Part print with two shaded views. Sizes in mm from the minimum x, y, z corner. A direction names the side the tool comes from. Give positions to 0.01 mm unless a question says otherwise; leave off trailing zeros. Order: outer loops, then holes, each group sorted by start corner. A loop starts at its lowest first (then second) coordinate and runs counter-clockwise, first axis right, second up. Notation, with made-up numbers: M 35.5,39 L 85.5,39 A12 ccw 85.5,51 Z; hole C -37.5,87.25 d9. An arc over 180 degrees is marked long. Return JSON: item names as keys, results as strings.
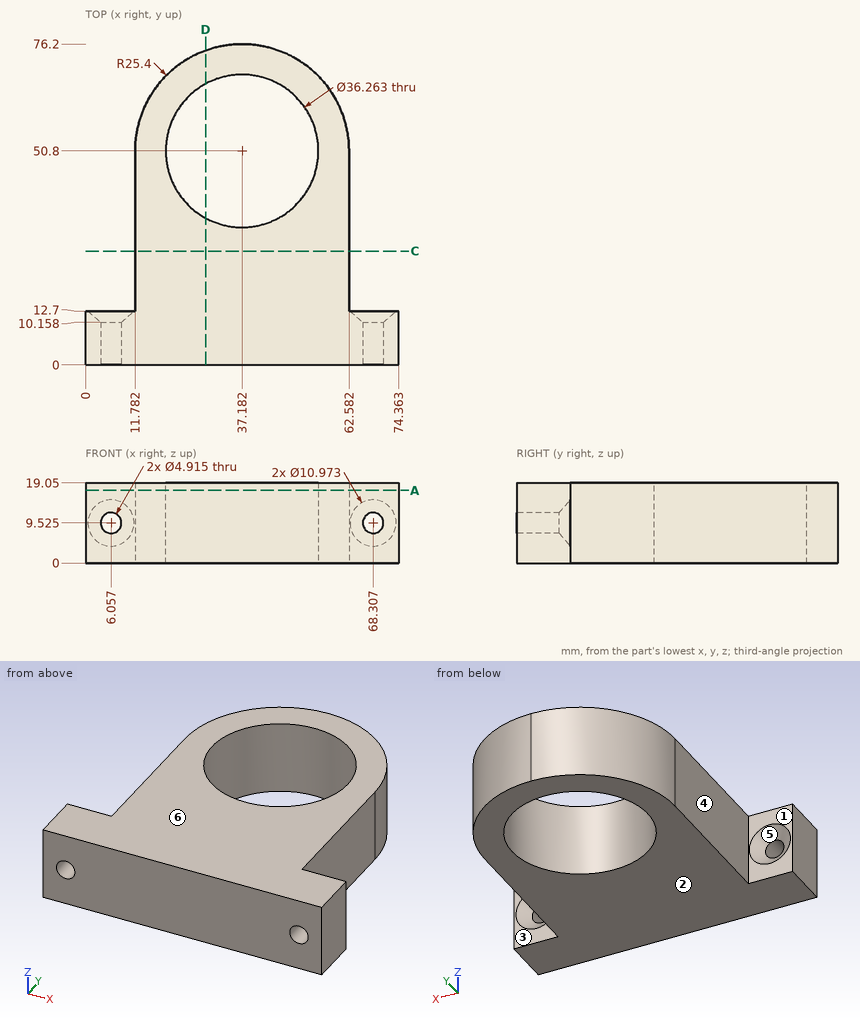
Q1. Probe line 1 along Y through (x, z) = (37, 2.5); line 2 along X through (y, z) = (12.5, 11.75) (1 decimal); line 3 along X through (y, z) = (31, 11.75). List the from-to ranges inside material, lowest first.
Established:
{"line 1": "y = 0 to 32.67, 68.93 to 76.2", "line 2": "x = 0 to 1.3, 10.8 to 63.6, 73.1 to 74.4", "line 3": "x = 11.78 to 62.58"}
Q2. 3-axis set-ups, long thin cutter, end or side, ignore diameter. For the marked faces 1, 2 and 3: which of +Z, -Z, +X, -X, +Y, -Y reach the whole face in a straight line?
Established:
{"face 1": "+Z, -Z, -X, +Y", "face 2": "-Z, +X, -X, +Y, -Y", "face 3": "+Z, -Z, +X, +Y"}
Q3. Band-saw the part on A-A (z = 17.25). Give the cut face in (x, y), then the cut area to 3 significant figures.
Established:
{"outline": "M 0,0 L 74.36,0 L 74.36,12.7 L 62.58,12.7 L 62.58,50.8 A25.4 ccw 11.78,50.8 L 11.78,12.7 L 0,12.7 Z; hole C 37.18,50.8 d36.26", "area": "2,860 mm²"}
Q4. Two-plate mould, pull along Z, no slides. Class the marked faces 4, 5 and 6: +Z half, -Z half, draft (parallel to the pull), parting line (faces both ways), or undercut.
Established:
{"face 4": "draft", "face 5": "undercut", "face 6": "+Z half"}
Q5. Pin check, flat tips, straight feed: pin 1 (10 mm diameter, centred on x = 34, y = 67, fed in from +Z); pin 2 (5.5 mm diameter, centred on x = 68.31, z = 9.53, fed in from +Y); pin 3 (2 mm diameter, centred on x = 64.5, y = 18.5, fed in from -Z); pin 4 (9.5 mm diameter, centred on x = 71, z = 7, fed in from +Y). Stop position of each tip, or through.
Established:
{"pin 1": "stops at z = 19.05", "pin 2": "stops at y = 10.41", "pin 3": "passes through", "pin 4": "stops at y = 12.7"}
Q6. Band-saw the part on D-D (x = 28.5). Give the cut face in (y, z).
Established:
{"outline": "M 0,0 L 34.88,0 L 34.88,19.05 L 0,19.05 Z; M 66.72,0 L 74.67,0 L 74.67,19.05 L 66.72,19.05 Z"}
Q7. Band-saw the part on C-C (y = 27). Give the cut face in (x, z).
Established:
{"outline": "M 11.78,0 L 62.58,0 L 62.58,19.05 L 11.78,19.05 Z"}
